from build123d import *

# Parameters (mm, degrees)
SKETCH1_R           = 101.6
BOSS_EXTRUDE1_DEPTH = 5.08
BOSS_EXTRUDE2_START = 25.4
SKETCH4_R           = 101.6
BOSS_EXTRUDE2_DEPTH = 25.4
SKETCH5_R           = 56.642
BOSS_EXTRUDE3_DEPTH = 12.7
CUT_EXTRUDE3_START  = -64.008
SKETCH6_R           = 56.642
CUT_EXTRUDE3_DEPTH  = 64.008
CUT_EXTRUDE6_START  = -25.4
SKETCH10_R          = 98.425
SKETCH10_R_2        = 56.642
CUT_EXTRUDE6_DEPTH  = 25.4
SKETCH16_R          = 3.175
CUT_EXTRUDE7_DEPTH  = 6.35
SKETCH17_R          = 3.175
CUT_EXTRUDE8_DEPTH  = 7.874


with BuildPart() as part:
    # Sketch1 → Boss-Extrude1 (new body)
    with BuildSketch(Plane.XY):
        Circle(SKETCH1_R)
    extrude(amount=BOSS_EXTRUDE1_DEPTH)

    # Sketch4 → Boss-Extrude2 (add)
    with BuildSketch(Plane(origin=(0, 0, 0), x_dir=(-1, 0, 0), z_dir=(0, 0, -1)).offset(BOSS_EXTRUDE2_START)):
        Circle(SKETCH4_R)
    extrude(amount=-BOSS_EXTRUDE2_DEPTH)

    # Sketch5 → Boss-Extrude3 (add)
    with BuildSketch(Plane(origin=(0, 0, -25.4), x_dir=(-1, 0, 0), z_dir=(0, 0, -1))):
        Circle(SKETCH5_R)
    extrude(amount=BOSS_EXTRUDE3_DEPTH)

    # Sketch6 → Cut-Extrude3 (cut)
    with BuildSketch(Plane(origin=(0, 0, -38.1), x_dir=(-1, 0, 0), z_dir=(0, 0, -1)).offset(CUT_EXTRUDE3_START)):
        Circle(SKETCH6_R)
    extrude(amount=CUT_EXTRUDE3_DEPTH, mode=Mode.SUBTRACT)

    # Sketch10 → Cut-Extrude6 (cut)
    with BuildSketch(Plane(origin=(0, 0, -25.4), x_dir=(-1, 0, 0), z_dir=(0, 0, -1)).offset(CUT_EXTRUDE6_START)):
        Circle(SKETCH10_R)
        Circle(SKETCH10_R_2, mode=Mode.SUBTRACT)
    extrude(amount=CUT_EXTRUDE6_DEPTH, mode=Mode.SUBTRACT)

    # Sketch16 → Cut-Extrude7 (cut)
    with BuildSketch(Plane(origin=(0, 0, 0), x_dir=(-1, 0, 0), z_dir=(0, 0, -1))):
        with Locations((53.848, 40.259)):
            Circle(SKETCH16_R)
        with Locations((-53.848, 40.259)):
            Circle(SKETCH16_R)
        with Locations((-53.848, -40.259)):
            Circle(SKETCH16_R)
        with Locations((53.848, -40.259)):
            Circle(SKETCH16_R)
    extrude(amount=-CUT_EXTRUDE7_DEPTH, mode=Mode.SUBTRACT)

    # Sketch17 → Cut-Extrude8 (cut)
    with BuildSketch(Plane.XY.offset(5.08)):
        with Locations((54.055769112, 74.294164254)):
            Circle(SKETCH17_R)
        with Locations((-53.640230888, 74.294164254)):
            Circle(SKETCH17_R)
        with Locations((-53.640230888, -74.295835746)):
            Circle(SKETCH17_R)
        with Locations((54.055769112, -74.295835746)):
            Circle(SKETCH17_R)
    extrude(amount=-CUT_EXTRUDE8_DEPTH, mode=Mode.SUBTRACT)


solid = part.part
CAD build for the part. Positions are in the model's coordinates, mm. A direction names the side the tool comes from. Round coordinates to 2 decimals unless told otherwise and drop trailing zeros. Order: outer loops, then holes, each group sorted by start corner. A loop starts at its lowest first (then second) coordinate and runs counter-clockwise, first axis right, second up. Notation, with made-up numbers: M -39.75,-19.75 L -20.75,-19.75 A9 cw -20.75,-13.75 Z; hole C 0,58 d5. An arc over 180 degrees is marked long. Use one line per item in the form item = value.
Q1. Saw through at C-C on x = 81. Give the cut face in (y, z).
Recorded:
outline = M -61.33,-25.4 L -55.91,-25.4 L -55.91,0 L 55.91,0 L 55.91,-25.4 L 61.33,-25.4 L 61.33,5.08 L -61.33,5.08 Z
Q2. Saw through at A-A on y = 0. Give the cut face in (x, z) (3 decimals).
Recorded:
outline = M -101.6,-25.4 L -98.425,-25.4 L -98.425,0 L -56.642,0 L -56.642,5.08 L -101.6,5.08 Z; M 56.642,0 L 98.425,0 L 98.425,-25.4 L 101.6,-25.4 L 101.6,5.08 L 56.642,5.08 Z
Q3. Which spindle directions (+Z, -Z, +X, -X, +Y, -Y) get a long thin tool onto all of the face, cutting with end or side? Do faces 3 (the cylindrical face through (-93.88, 29.56, -12.52)), 4 (the cylindrical face through (-55.98, -72.15, 2.58)). Say none if no direction does.
Recorded:
face_3 = -Z
face_4 = +Z, -Z
Q4. Probe L1, parallel to Y at x = 0, z = 2; L2, parallel to Y at x = 1, z = -6. List the from-to ranges inside material, lowest first.
Recorded:
L1 = -101.6 to -56.64, 56.64 to 101.6
L2 = -101.6 to -98.42, 98.42 to 101.6
Q5. Flat gauge pins, fed straight in: P1, Ø1, axis at x = -56, y = 2, coming from the -Z side; P2, Ø12, axis at x = -54, z = -7, coming from the -Y side; P3, Ø3, axis at y = 79.5, z = -13.5, coming from the +X side; P4, Ø8, axis at x = -77, y = 33.5, coming from the -Z side. Where does each tip first touch, or does it go through?
Recorded:
P1 = through
P2 = -89.55
P3 = 65.1
P4 = 0
Q6. Two-plate mould, pull along Y, no slides. Class faces 1 (the flat face through (83.3, 53.2, -25.4)), 2 (the cylindrical face through (7.37, 56.16, 2.58)): +Y half, -Y half, draft (parallel to the pull), parting line (faces both ways), or undercut.
Recorded:
face_1 = draft
face_2 = undercut
Q7. Saw through at D-D on z = -5.5. Give the cut face in (x, y) (3 decimals), then the cut area to 3 significant figures.
Recorded:
outline = C 0,0 d203.2; hole C 0,0 d196.85
area = 2,000 mm^2
